Read the model definition and answer for the solid it produces. Units are mm, in the model's axes. Face numbers are marked on the shaded views. A direction names the side the tool comes from. Round coordinates to 2 decimals unless told otherwise and drop trailing zeros. Write each loop counter-clockwise with the first axis right and the second up, starting at its lowest first coordinate (ties: lowest second). Pieces come first, ordered by that corner, then holes. Notation, with made-up numbers: (-18, 21) -> (26, 21) arc R15 ccw to (26, 33) -> close; hole circle Ø7 at (49, 0.5). An arc over 180 degrees is marked (long way). Return JSON: item names as keys, results as strings. Group by question number.
(1) A cutting plane is placed at D-D on y = -6. Give the vertices of the cut face in (x, z).
(2) A cutting plane is placed at B-B on y = -17. State how many separate pieces and enclosed holes the cut face has, then the cut area to 3 significant figures.
(3) A cutting plane is placed at A-A on z = 20. Give the vertices of the cut face in (x, y), then the cut area to 3 significant figures.
(4) Straight lines are drawn through the part: line 1 (Y direction, x = 15, z = 3.25); line 2 (X direction, y = 5, z = 13.5); line 3 (Y direction, x = -5, z = 19.5). For each, find the intervals that lie inside material, in ascending order.
(5) Given pin 1 (2 mm diameter, centred on x = -2, y = -10.5, fed in from +Z); pin 2 (1.5 mm diameter, centred on y = -17, z = 41.5, fed in from +X); pin 3 (11.5 mm diameter, centred on x = -1, y = 7.5, fed in from +Z); pin 4 (4.5 mm diameter, centred on y = -16.5, z = 11, fed in from -X), each flat-ended and moving along its own axis, determine where each tip first touches the part or whether it passes through.
(6) The mould has two halves that part along X. Classify the marked faces 4, 5, 6 and 7: released by +X, released by -X, zero draft, split by the parting line, or undercut.
(7) A cutting plane is placed at C-C on z = 14. Give the vertices of the cut face in (x, y), then the cut area to 3 significant figures.
(8) For the marked faces 1, 2 and 3, determine the directions among +Z, -Z, +X, -X, +Y, -Y from which every point of the face is accessible in a straight line to the end or side of a thin tool.
```python
from build123d import *

# Parameters (mm, degrees)
SKETCH1_W           = 41
SKETCH1_H           = 50.6
BOSS_EXTRUDE1_DEPTH = 6
FILLET1_R           = 3
SKETCH3_R           = 1.25
CUT_EXTRUDE1_DEPTH  = 34.111025354
SKETCH4_R           = 1.5
CUT_EXTRUDE2_DEPTH  = 0.5
SKETCH5_W           = 24.5
SKETCH5_H           = 46
CUT_EXTRUDE3_DEPTH  = 2.77
SKETCH6_W           = 6
SKETCH6_H           = 16
CUT_EXTRUDE4_DEPTH  = 1.5
SKETCH7_W           = 23
SKETCH7_H           = 48.75
SKETCH7_W_2         = 13
SKETCH7_H_2         = 4.000096304
BOSS_EXTRUDE2_DEPTH = 10
SKETCH8_W           = 23
SKETCH8_H           = 4
BOSS_EXTRUDE3_DEPTH = 44
SKETCH9_R           = 1
CUT_EXTRUDE5_DEPTH  = 82.120959067


with BuildPart() as part:
    # Sketch1 → Boss-Extrude1 (new body)
    with BuildSketch(Plane.XY):
        Rectangle(SKETCH1_W, SKETCH1_H)
    extrude(amount=BOSS_EXTRUDE1_DEPTH)

    # Fillet1
    fillet1_edges = [part.edges().sort_by_distance(p)[0] for p in [
        (20.5, -25.3, 3),
        (-20.5, -25.3, 3),
        (-20.5, 25.3, 3),
        (20.5, 25.3, 3),
    ]]
    fillet(fillet1_edges, radius=FILLET1_R)

    # Sketch3 → Cut-Extrude1 (cut, through all)
    with BuildSketch(Plane.XY.offset(6)):
        with Locations((-15, 0)):
            Circle(SKETCH3_R)
        with Locations((-15, 17)):
            Circle(SKETCH3_R)
        with Locations((-15, -17)):
            Circle(SKETCH3_R)
    cut_extrude1 = extrude(amount=-CUT_EXTRUDE1_DEPTH, mode=Mode.SUBTRACT)

    # Mirror1: Cut-Extrude1 across plane
    add(cut_extrude1.mirror(Plane(origin=(0, 0, 0), x_dir=(0, 0, 1), z_dir=(1, 0, 0))), mode=Mode.SUBTRACT)

    # Sketch4 → Cut-Extrude2 (cut)
    with BuildSketch(Plane.XY.offset(6)):
        with Locations((-15, 17)):
            Circle(SKETCH4_R)
        with Locations((-15, 0)):
            Circle(SKETCH4_R)
        with Locations((-15, -17)):
            Circle(SKETCH4_R)
    cut_extrude2 = extrude(amount=-CUT_EXTRUDE2_DEPTH, mode=Mode.SUBTRACT)

    # Mirror2: Cut-Extrude2 across plane
    add(cut_extrude2.mirror(Plane(origin=(0, 0, 0), x_dir=(0, 0, 1), z_dir=(1, 0, 0))), mode=Mode.SUBTRACT)

    # Sketch5 → Cut-Extrude3 (cut)
    with BuildSketch(Plane(origin=(0, 0, 0), x_dir=(-1, 0, 0), z_dir=(0, 0, -1))):
        with Locations((0, 2.3)):
            Rectangle(SKETCH5_W, SKETCH5_H)
    extrude(amount=-CUT_EXTRUDE3_DEPTH, mode=Mode.SUBTRACT)

    # Sketch6 → Cut-Extrude4 (cut)
    with BuildSketch(Plane(origin=(0, 0, 2.77), x_dir=(-1, 0, 0), z_dir=(0, 0, -1))):
        with Locations((0, 17.3)):
            Rectangle(SKETCH6_W, SKETCH6_H)
    extrude(amount=-CUT_EXTRUDE4_DEPTH, mode=Mode.SUBTRACT)

    # Sketch7 → Boss-Extrude2 (add)
    with BuildSketch(Plane.XY.offset(6)):
        with Locations((0, 0.925)):
            Rectangle(SKETCH7_W, SKETCH7_H)
        with Locations((0, 11.300440592)):
            Rectangle(SKETCH7_W_2, SKETCH7_H_2, mode=Mode.SUBTRACT)
        with Locations((0, 18.300440592)):
            Rectangle(SKETCH7_W_2, SKETCH7_H_2, mode=Mode.SUBTRACT)
        with Locations((0, 4.300440592)):
            Rectangle(SKETCH7_W_2, SKETCH7_H_2, mode=Mode.SUBTRACT)
        with Locations((0, -2.699559408)):
            Rectangle(SKETCH7_W_2, SKETCH7_H_2, mode=Mode.SUBTRACT)
        with Locations((0, -9.699559408)):
            Rectangle(SKETCH7_W_2, SKETCH7_H_2, mode=Mode.SUBTRACT)
        with Locations((0, -16.699559408)):
            Rectangle(SKETCH7_W_2, SKETCH7_H_2, mode=Mode.SUBTRACT)
    extrude(amount=BOSS_EXTRUDE2_DEPTH)

    # Sketch8 → Boss-Extrude3 (add)
    with BuildSketch(Plane.XY.offset(16)):
        with Locations((0, 23.3)):
            Rectangle(SKETCH8_W, SKETCH8_H)
        with Locations((0, -21.45)):
            Rectangle(SKETCH8_W, SKETCH8_H)
    extrude(amount=BOSS_EXTRUDE3_DEPTH)

    # Sketch9 → Cut-Extrude5 (cut, through all)
    with BuildSketch(Plane(origin=(0, 25.3, 0), x_dir=(1, 0, 0), z_dir=(0, 1, 0))):
        with BuildLine():
            Line((11.5, -60), (11.5, -37))
            ThreePointArc((11.5, -37), (0, -48.5), (-11.5, -37))
            Line((-11.5, -37), (-11.5, -60))
            Line((-11.5, -60), (11.5, -60))
        make_face()
        with BuildLine():
            ThreePointArc((-4, -37), (0, -41), (4, -37))
            Line((4, -37), (-4, -37))
        make_face()
        with BuildLine():
            Line((-4, -37), (4, -37))
            ThreePointArc((4, -37), (0, -33), (-4, -37))
        make_face()
        with Locations(Location((0, -29, 0), (0, 0, 180))):
            Circle(SKETCH9_R)
        with Locations(Location((-5.656854249, -31.343145751, 0), (0, 0, 180))):
            Circle(SKETCH9_R)
        with BuildLine():
            ThreePointArc((-7, -37), (-8, -36), (-9, -37))
            Line((-9, -37), (-7, -37))
        make_face()
        with BuildLine():
            Line((-7, -37), (-9, -37))
            ThreePointArc((-9, -37), (-8, -38), (-7, -37))
        make_face()
        with Locations(Location((-5.656854249, -42.656854249, 0), (0, 0, 180))):
            Circle(SKETCH9_R)
        with Locations(Location((0, -45, 0), (0, 0, 180))):
            Circle(SKETCH9_R)
        with Locations(Location((5.656854249, -42.656854249, 0), (0, 0, 180))):
            Circle(SKETCH9_R)
        with BuildLine():
            ThreePointArc((7, -37), (8, -38), (9, -37))
            Line((9, -37), (7, -37))
        make_face()
        with BuildLine():
            Line((7, -37), (9, -37))
            ThreePointArc((9, -37), (8, -36), (7, -37))
        make_face()
        with Locations(Location((5.656854249, -31.343145751, 0), (0, 0, 180))):
            Circle(SKETCH9_R)
    extrude(amount=-CUT_EXTRUDE5_DEPTH, mode=Mode.SUBTRACT)


solid = part.part
```
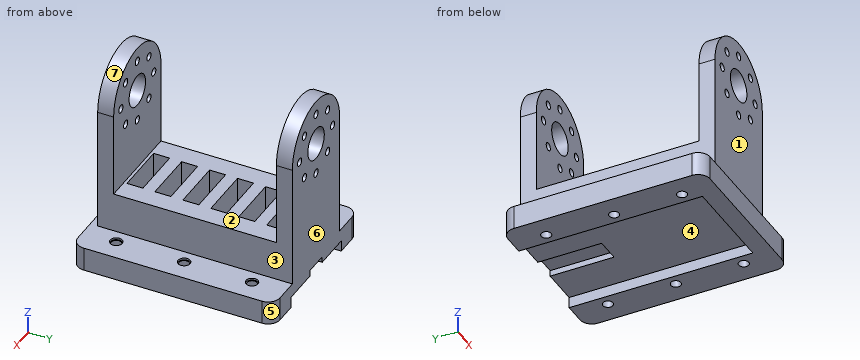
Checks:
{
 "1": {"outline": "(-20.5, 0) -> (-12.25, 0) -> (-12.25, 2.77) -> (12.25, 2.77) -> (12.25, 0) -> (20.5, 0) -> (20.5, 6) -> (11.5, 6) -> (11.5, 16) -> (-11.5, 16) -> (-11.5, 6) -> (-20.5, 6) -> close"},
 "2": {"separate pieces": "3", "enclosed holes": "0", "area": "248 mm^2"},
 "3": {"outline": "(-11.5, -23.45) -> (11.5, -23.45) -> (11.5, -19.45) -> (-11.5, -19.45) -> close; (-11.5, 21.3) -> (11.5, 21.3) -> (11.5, 25.3) -> (-11.5, 25.3) -> close", "area": "184 mm^2"},
 "4": {"line 1": "y = -25.3 to -18.25, -15.75 to -1.25, 1.25 to 15.75, 18.25 to 25.3", "line 2": "x = -11.5 to -6.5, 6.5 to 11.5", "line 3": "y = -23.45 to -19.45, 21.3 to 25.3"},
 "5": {"pin 1": "stops at z = 6", "pin 2": "passes through", "pin 3": "stops at z = 16", "pin 4": "stops at x = -11.5"},
 "6": {"face 4": "undercut", "face 5": "released by +X", "face 6": "zero draft", "face 7": "split by the parting line"},
 "7": {"outline": "(-11.5, -23.45) -> (11.5, -23.45) -> (11.5, 25.3) -> (-11.5, 25.3) -> close; hole (-6.5, -18.7) -> (6.5, -18.7) -> (6.5, -14.7) -> (-6.5, -14.7) -> close; hole (-6.5, -11.7) -> (6.5, -11.7) -> (6.5, -7.7) -> (-6.5, -7.7) -> close; hole (-6.5, -4.7) -> (6.5, -4.7) -> (6.5, -0.7) -> (-6.5, -0.7) -> close; hole (-6.5, 2.3) -> (6.5, 2.3) -> (6.5, 6.3) -> (-6.5, 6.3) -> close; hole (-6.5, 9.3) -> (6.5, 9.3) -> (6.5, 13.3) -> (-6.5, 13.3) -> close; hole (-6.5, 16.3) -> (6.5, 16.3) -> (6.5, 20.3) -> (-6.5, 20.3) -> close", "area": "809 mm^2"},
 "8": {"face 1": "+Z, +X, -X, -Y", "face 2": "+Z, +X, -X", "face 3": "+Z, +X, +Y, -Y"}
}
